For this review, take the finished solid that the model builds, in its own axes (mm). Face numbers are marked on the shaded views. A direction names the side the tool comes from. Give positions to 0.01 mm unless a question says otherwise; leave off trailing zeros. Loops run counter-clockwise (first coordinate to the right, second up) from the corner with the lowest first, then second, coordinate; pieces in that order, holes last. Notation, with made-up numbers: (-8.5, 13) - (16.5, 13) arc R30 ccw to (16.5, 51) - close; hole circle Ø8 at (67, 65.5). An arc over 180 degrees is marked (long way). Put each result on its own line as item: value.
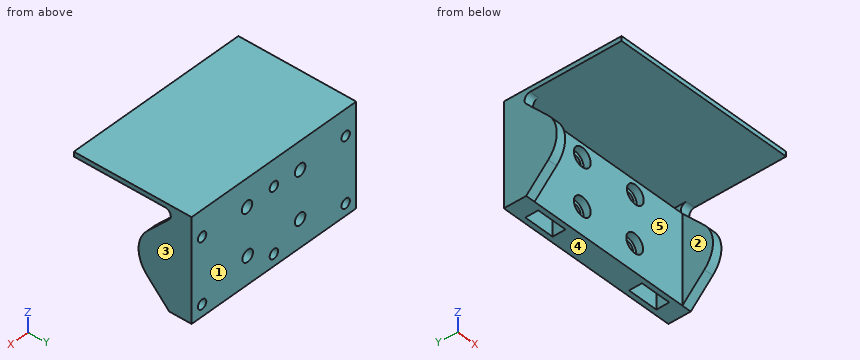
from build123d import *

# Parameters (mm, degrees)
SKETCH1_W           = 78.5
SKETCH1_H           = 37.4
BOSS_EXTRUDE1_DEPTH = 9.5
SKETCH6_R           = 2
CUT_EXTRUDE1_DEPTH  = 6.5
BOSS_EXTRUDE2_DEPTH = 4
SKETCH9_W           = 13
SKETCH9_H           = 5.5
CUT_EXTRUDE3_DEPTH  = 56.75233179
BOSS_EXTRUDE3_REACH = 83.737
BOSS_EXTRUDE4_START = -4
BOSS_EXTRUDE4_DEPTH = 4
BOSS_EXTRUDE5_DEPTH = 4
SKETCH15_R          = 2.5
CUT_EXTRUDE4_DEPTH  = 15
SKETCH16_R          = 4
CUT_EXTRUDE5_DEPTH  = 3


with BuildPart() as part:
    # Sketch1 → Boss-Extrude1 (new body)
    with BuildSketch(Plane(origin=(0, 0, 0), x_dir=(1, 0, 0), z_dir=(0, 1, 0))):
        Rectangle(SKETCH1_W, SKETCH1_H)
    extrude(amount=BOSS_EXTRUDE1_DEPTH)

    # Sketch6 → Cut-Extrude1 (cut)
    with BuildSketch(Plane(origin=(0, 9.5, 0), x_dir=(1, 0, 0), z_dir=(0, 1, 0))):
        with Locations(Location((-34.25, 13.7, 0), (0, 0, 270))):
            Circle(SKETCH6_R)
        with Locations(Location((0, 13.7, 0), (0, 0, 270))):
            Circle(SKETCH6_R)
        with Locations(Location((34.25, 13.7, 0), (0, 0, 270))):
            Circle(SKETCH6_R)
        with Locations(Location((34.25, -13.7, 0), (0, 0, 270))):
            Circle(SKETCH6_R)
        with Locations(Location((0, -13.7, 0), (0, 0, 270))):
            Circle(SKETCH6_R)
        with Locations(Location((-34.25, -13.7, 0), (0, 0, 270))):
            Circle(SKETCH6_R)
    extrude(amount=-CUT_EXTRUDE1_DEPTH, mode=Mode.SUBTRACT)

    # Sketch7 → Boss-Extrude2 (add)
    with BuildSketch(Plane.ZY.offset(39.25)):
        with BuildLine():
            Line((-18.7, 0), (-9.037433155, -9.344774046))
            ThreePointArc((-9.037433155, -9.344774046), (0, -13), (9.037433155, -9.344774046))
            Line((9.037433155, -9.344774046), (18.7, 0))
            Line((18.7, 0), (-18.7, 0))
        make_face()
    boss_extrude2 = extrude(amount=-BOSS_EXTRUDE2_DEPTH)

    # Mirror1: Boss-Extrude2 across plane
    add(boss_extrude2.mirror(Plane(origin=(0, 0, 0), x_dir=(0, 0, 1), z_dir=(1, 0, 0))))

    # Sketch9 → Cut-Extrude3 (cut, through all)
    with BuildSketch(Plane(origin=(0, 0, -18.7), x_dir=(-1, 0, 0), z_dir=(0, 0, -1))):
        with Locations((24.75, 4.75)):
            Rectangle(SKETCH9_W, SKETCH9_H)
        with Locations((-24.75, 4.75)):
            Rectangle(SKETCH9_W, SKETCH9_H)
    extrude(amount=-CUT_EXTRUDE3_DEPTH, mode=Mode.SUBTRACT)

    # Boss-Extrude3: up to this face of the body (flat: up to its plane)
    boss_extrude3_end = Plane(part.part.faces().sort_by_distance((39.25, 0.189608499, 0))[0])
    # Sketch11 → Boss-Extrude3 (add, up to the picked face)
    with BuildSketch(Plane.ZY.offset(39.25), mode=Mode.PRIVATE) as boss_extrude3_sk1:
        with BuildLine():
            Line((18.7, 9.5), (24.7, 9.5))
            Line((24.7, 9.5), (24.7, -40.5))
            Line((24.7, -40.5), (22.7, -40.5))
            Line((22.7, -40.5), (22.7, 3.5))
            ThreePointArc((22.7, 3.5), (21.528427125, 6.328427125), (18.7, 7.5))
            Line((18.7, 7.5), (18.7, 9.5))
        make_face()
    boss_extrude3_tool1 = split(extrude(boss_extrude3_sk1.sketch, amount=-BOSS_EXTRUDE3_REACH, mode=Mode.PRIVATE), bisect_by=boss_extrude3_end, keep=Keep.BOTH, mode=Mode.PRIVATE)
    add(boss_extrude3_tool1.solids().sort_by(Axis((-39.25, -13.095828, 23.426281), (1, 0, 0)))[0])

    # Sketch12 → Boss-Extrude4 (add)
    with BuildSketch(Plane(origin=(39.25, 0, 0), x_dir=(0, 0, -1), z_dir=(1, 0, 0)).offset(BOSS_EXTRUDE4_START)):
        with BuildLine():
            Line((-18.7, 7.5), (-18.7, 0))
            ThreePointArc((-18.7, 0), (-21.261557408, 0.476218058), (-22.7, -1.696163792))
            Line((-22.7, -1.696163792), (-22.7, 3.5))
            ThreePointArc((-22.7, 3.5), (-21.528427125, 6.328427125), (-18.7, 7.5))
        make_face()
    extrude(amount=BOSS_EXTRUDE4_DEPTH)

    # Sketch13 → Boss-Extrude5 (add)
    with BuildSketch(Plane.ZY.offset(39.25)):
        with BuildLine():
            Line((22.7, -1.696163792), (22.7, 3.5))
            ThreePointArc((22.7, 3.5), (21.528427125, 6.328427125), (18.7, 7.5))
            Line((18.7, 7.5), (18.7, 0))
            ThreePointArc((18.7, 0), (21.261557408, 0.476218058), (22.7, -1.696163792))
        make_face()
    extrude(amount=-BOSS_EXTRUDE5_DEPTH)

    # Sketch15 → Cut-Extrude4 (cut)
    with BuildSketch(Plane(origin=(0, 9.5, 0), x_dir=(1, 0, 0), z_dir=(0, 1, 0))):
        with Locations(Location((-12.5, 7, 0), (0, 0, 270))):
            Circle(SKETCH15_R)
        with Locations(Location((-12.5, -13, 0), (0, 0, 270))):
            Circle(SKETCH15_R)
        with Locations(Location((12.816690271, -13, 0), (0, 0, 270))):
            Circle(SKETCH15_R)
        with Locations(Location((12.5, 7, 0), (0, 0, 270))):
            Circle(SKETCH15_R)
    extrude(amount=-CUT_EXTRUDE4_DEPTH, mode=Mode.SUBTRACT)

    # Sketch16 → Cut-Extrude5 (cut)
    with BuildSketch(Plane.XZ):
        with Locations(Location((-12.5, 13, 0), (0, 0, 270))):
            Circle(SKETCH16_R)
        with Locations(Location((12.816690271, 13, 0), (0, 0, 270))):
            Circle(SKETCH16_R)
        with Locations(Location((12.5, -7, 0), (0, 0, 270))):
            Circle(SKETCH16_R)
        with Locations(Location((-12.5, -7, 0), (0, 0, 270))):
            Circle(SKETCH16_R)
    extrude(amount=-CUT_EXTRUDE5_DEPTH, mode=Mode.SUBTRACT)


solid = part.part
1) Take a section at A-A on x = -12.5. State the section outline as (y, z) points.
Geometry check:
outline: (-40.5, 22.7) - (3.5, 22.7) arc R4 cw to (7.5, 18.7) - (0, 18.7) - (0, 17) - (3, 17) - (3, 15.5) - (9.5, 15.5) - (9.5, 24.7) - (-40.5, 24.7) - close; (0, -18.7) - (9.5, -18.7) - (9.5, -9.5) - (3, -9.5) - (3, -11) - (0, -11) - close; (0, -3) - (3, -3) - (3, -4.5) - (9.5, -4.5) - (9.5, 10.5) - (3, 10.5) - (3, 9) - (0, 9) - close
2) Take a section at D-D on x = 0. State the section outline as (y, z) points, and give its area (3 significant figures).
Geometry check:
outline: (-40.5, 22.7) - (3.5, 22.7) arc R4 cw to (7.5, 18.7) - (0, 18.7) - (0, -18.7) - (9.5, -18.7) - (9.5, -15.7) - (3, -15.7) - (3, -11.7) - (9.5, -11.7) - (9.5, 11.7) - (3, 11.7) - (3, 15.7) - (9.5, 15.7) - (9.5, 24.7) - (-40.5, 24.7) - close
area: 415 mm²
3) Wall thickness on line 1 (X direction, y = 1, z = -7); line 2 (X direction, y = 5, z = -1); line 3 (Z direction, x = -35, y = 1): over which ranges is each line inside the solid? List them lowest first.
Geometry check:
line 1: x = -39.25 to -16.5, -8.5 to 8.5, 16.5 to 39.25
line 2: x = -39.25 to -31.25, -18.25 to 18.25, 31.25 to 39.25
line 3: z = -18.7 to 18.7, 22.7 to 24.7
4) Take a section at C-C on z = -6. State how many separate pieces and enclosed holes the cut face has, and give its area (3 significant figures).
Geometry check:
separate pieces: 3
enclosed holes: 2
area: 589 mm²
5) Draft analysis for pull direction X (two halves, no side actions). For the marked faces 1, 2 and 3, state which applies: pulls with the +X half, pulls with the -X half, needs draft (parallel to the pull), parting line crosses it, or undercut.
Geometry check:
face 1: needs draft
face 2: undercut
face 3: pulls with the +X half
6) Take a section at B-B on x = 23. State the section outline as (y, z) points.
Geometry check:
outline: (-40.5, 22.7) - (3.5, 22.7) arc R4 cw to (7.5, 18.7) - (7.5, -18.7) - (9.5, -18.7) - (9.5, 24.7) - (-40.5, 24.7) - close; (0, -18.7) - (2, -18.7) - (2, 18.7) - (0, 18.7) - close
7) For the marked faces 4 and 5, list the 3-axis set-ups (+Z, -Z, +X, -X, +Y, -Y) from which the entire face can be reached by the end or side of a thin tool; tool diameter is ignored.
Geometry check:
face 4: -Z, +X, -X, +Y, -Y
face 5: -Z, -Y
8) Insertion check: pin 1 Ø8 at (x, y) = (10, -21.5) entering from -Z; pin 2 Ø6.5 at (x, z) = (-11, 14) entering from -Y; pin 3 Ø3 at (x, z) = (-12.5, 13) entering from +Y; pin 4 Ø6.5 at (x, z) = (-12.5, 13) entering from -Y. Each pin has a flat end and moves straight along its axis. Give the tip position at first contact, or say it passes through.
Geometry check:
pin 1: stops at z = 22.7
pin 2: stops at y = 0
pin 3: passes through
pin 4: stops at y = 3
